```python
from build123d import *

# Parameters (mm, degrees)
EXTRUDE_1_DEPTH          = 5
FILLET_1_R               = 2
CUT_EXTRUDE_1_DEPTH      = 57.259132592
CUT_EXTRUDE_1_DEPTH_BACK = 57.259132592


with BuildPart() as part:
    # 草图1 → 凸台-拉伸1 (new body)
    with BuildSketch(Plane(origin=(0, 0, 0), x_dir=(1, 0, 0), z_dir=(0, 1, 0))):
        Polygon((25.3, -50), (25.3, 17), (-25.3, 17), (-25.3, -50), (-0.631149451, -50), (0.631149451, -50), align=None)
        with BuildLine():
            ThreePointArc((-13.3, -40), (-15.3, -42), (-17.3, -40))
            ThreePointArc((-17.3, -40), (-15.3, -38), (-13.3, -40))
        make_face(mode=Mode.SUBTRACT)
        with BuildLine():
            ThreePointArc((13.3, -40), (15.3, -38), (17.3, -40))
            ThreePointArc((17.3, -40), (15.3, -42), (13.3, -40))
        make_face(mode=Mode.SUBTRACT)
    extrude(amount=EXTRUDE_1_DEPTH)

    # 圆角1
    fillet_1_edges = [part.edges().sort_by_distance(p)[0] for p in [
        (25.3, 2.5, 50),
        (-25.3, 2.5, 50),
        (-25.3, 2.5, -17),
        (25.3, 2.5, -17),
    ]]
    fillet(fillet_1_edges, radius=FILLET_1_R)

    # 草图2 → 切除-拉伸1 (cut, two sides: drawn at the far end of the back side and taken through both)
    with BuildSketch(Plane(origin=(0, 5, 0), x_dir=(1, 0, 0), z_dir=(0, 1, 0)).offset(-CUT_EXTRUDE_1_DEPTH_BACK)):
        with BuildLine():
            Line((20, 8.678912506), (20, -31.321087494))
            ThreePointArc((20, -31.321087494), (18, -33.321087494), (16, -31.321087494))
            Line((16, -31.321087494), (16, 8.678912506))
            ThreePointArc((16, 8.678912506), (18, 10.678912506), (20, 8.678912506))
        make_face()
        with BuildLine():
            Line((-20, 8.678912506), (-20, -31.321087494))
            ThreePointArc((-20, -31.321087494), (-18, -33.321087494), (-16, -31.321087494))
            Line((-16, -31.321087494), (-16, 8.678912506))
            ThreePointArc((-16, 8.678912506), (-18, 10.678912506), (-20, 8.678912506))
        make_face()
    extrude(amount=CUT_EXTRUDE_1_DEPTH + CUT_EXTRUDE_1_DEPTH_BACK, mode=Mode.SUBTRACT)


solid = part.part
```
Read the model definition and answer for the solid it produces. Units are mm, in the model's axes. A direction names the side the tool comes from. Coordinates: 2 decimals unless noted, no trailing zeros. Loops run counter-clockwise (first coordinate to the right, second up) from the corner with the lowest first, then second, coordinate; pieces in that order, holes last.
(1) The part is cut by section D-D (x = 18). Determine the outline of the cut face in (y, z), and give its area (3 significant figures).
Solution:
outline: (0, -17) - (5, -17) - (5, -10.68) - (0, -10.68) - close; (0, 33.32) - (5, 33.32) - (5, 50) - (0, 50) - close
area: 115 mm2
(2) A flat-ended cylindrical pin translates along its axis: pin 1 Ø5 at (x, z) = (-18, -6) entering from -Y. Find the tip coordinate at first contact, or state that the pin passes through.
Solution:
pin 1: stops at y = 0
(3) The part is cut by section B-B (y = 2). Determine the outline of the cut face in (x, z).
Solution:
outline: (-25.3, -15) arc R2 ccw to (-23.3, -17) - (23.3, -17) arc R2 ccw to (25.3, -15) - (25.3, 48) arc R2 ccw to (23.3, 50) - (-23.3, 50) arc R2 ccw to (-25.3, 48) - close; hole (-20, -8.68) arc R2 ccw to (-16, -8.68) - (-16, 31.32) arc R2 ccw to (-20, 31.32) - close; hole circle Ø4 at (-15.3, 40); hole circle Ø4 at (15.3, 40); hole (16, -8.68) arc R2 ccw to (20, -8.68) - (20, 31.32) arc R2 ccw to (16, 31.32) - close
(4) The part is cut by section C-C (x = -15.3). Determine the outline of the cut face in (y, z).
Solution:
outline: (0, -17) - (5, -17) - (5, 38) - (0, 38) - close; (0, 42) - (5, 42) - (5, 50) - (0, 50) - close
(5) A tool of negligible diameter and unlimited length cuts with its end or side. For faces 4 (the face through (18.04, 2.47, 33.32)), 5 (the face through (-24.7, 2.54, 49.43)), from which of +Z, -Z, +X, -X, +Y, -Y can it reach the whole face along a straight path? Write none if from no direction.
Solution:
face 4: +Y, -Y
face 5: +Z, -X, +Y, -Y
(6) Consider line 1 along X through (y, z) = (0.85, 2); line 2 along Z through (x, y) = (15.3, 3.9); line 3 along Z through (x, y) = (-17.5, 1.7). Determine where each line is inside the solid, lowest interval first.
Solution:
line 1: x = -25.3 to -20, -16 to 16, 20 to 25.3
line 2: z = -17 to 38, 42 to 50
line 3: z = -17 to -10.62, 33.26 to 50
(7) The part is cut by section A-A (z = 20). Determine the outline of the cut face in (x, y).
Solution:
outline: (-25.3, 0) - (-20, 0) - (-20, 5) - (-25.3, 5) - close; (-16, 0) - (16, 0) - (16, 5) - (-16, 5) - close; (20, 0) - (25.3, 0) - (25.3, 5) - (20, 5) - close
(8) The mould has two halves that part along Z. Classify faces 1 (the face through (0, 2, -17)), 2 (the face through (16, 2, 12)), 3 (the face through (25.3, 2, 17)): released by +Z, released by -Z, zero draft, split by the parting line, or undercut.
Solution:
face 1: released by -Z
face 2: undercut
face 3: zero draft
